Geometry check sheet. Reference: the model listing, model coordinates, mm. Face numbers are marked on the shaded views. A direction names the side the tool comes from. Give positions to 0.01 mm unless a question says otherwise; leave off trailing zeros. Write each loop counter-clockwise with the first axis right and the second up, starting at its lowest first coordinate (ties: lowest second). Pieces come first, ordered by that corner, then holes.
(1) Cross-section at A-A (y = -72.5). Record the boundary of the cut face in (x, z).
(2) Mould release check, pull along Z, two halves, no side actions. Record for the marked faces 1, 2 and 3: +Z half, -Z half, draft (parallel to the pull), parting line (faces both ways), or undercut.
(3) Cross-section at C-C (z = 7.75). Record the boundary of the cut face in (x, y), and give its area (3 significant figures).
(4) Thickness scan on line 1 along Z through (x, y) = (4, -66); line 2 along X through (y, z) = (8, 4.75); line 3 along X through (y, z) = (-44, 12.5). Record the ranges inside material, lowest first.
(5) Tool access check on the marked faces 4, 5 and 6. Record the directions out of +Z, -Z, +X, -X, +Y, -Y that give a thin tool (end or side, any length) a straight path to the whole face; none if there is none.
(6) Depth check by flat-ended pin: P1, Ø2, axis at y = -72.5, z = 15.5, coming from the -X side; P2, Ø5, axis at x = 2, y = -75, coming from the -Z side; P3, Ø4, axis at x = 7.5, z = 14, coming from the -Y side; P4, Ø8, axis at x = -2, z = 10.5, coming from the -Y side. Enter the tip coordinate at first touch or a pass-through.
(7) Cross-section at B-B (y = 0). Record the boundary of the cut face in (x, z).
(8) Cross-section at D-D (z = 17.75). Record the boundary of the cut face in (x, y).
```python
from build123d import *

# Parameters (mm, degrees)
SKETCH1_R           = 10
BOSS_EXTRUDE1_DEPTH = 20
SKETCH2_W           = 10
SKETCH2_H           = 35
CUT_EXTRUDE1_DEPTH  = 10


with BuildPart() as part:
    # Sketch1 → Boss-Extrude1 (new body)
    with BuildSketch(Plane.XY):
        with BuildLine():
            Line((5, -42), (10, -42))
            ThreePointArc((10, -42), (15.132819854, -26.12111797), (29.113715132, -17.009625152))
            ThreePointArc((29.113715132, -17.009625152), (42.376973847, 2.071419783), (25, 17.5))
            ThreePointArc((25, 17.5), (0, 10.405357444), (-25, 17.5))
            ThreePointArc((-25, 17.5), (-42.376973847, 2.071419783), (-29.113715132, -17.009625152))
            ThreePointArc((-29.113715132, -17.009625152), (-15.132819854, -26.12111797), (-10, -42))
            Line((-10, -42), (-5, -42))
            Line((-5, -42), (-5, -87))
            Line((-5, -87), (5, -87))
            Line((5, -87), (5, -42))
        make_face()
        with Locations((-25, 0)):
            Circle(SKETCH1_R, mode=Mode.SUBTRACT)
        with Locations(Location((25, 0, 0), (0, 0, 180))):
            Circle(SKETCH1_R, mode=Mode.SUBTRACT)
    extrude(amount=BOSS_EXTRUDE1_DEPTH)

    # Sketch2 → Cut-Extrude1 (cut)
    with BuildSketch(Plane(origin=(5, 0, 0), x_dir=(0, 0, -1), z_dir=(1, 0, 0))):
        with Locations((-10, -69.5)):
            Rectangle(SKETCH2_W, SKETCH2_H)
    extrude(amount=-CUT_EXTRUDE1_DEPTH, mode=Mode.SUBTRACT)


solid = part.part
```
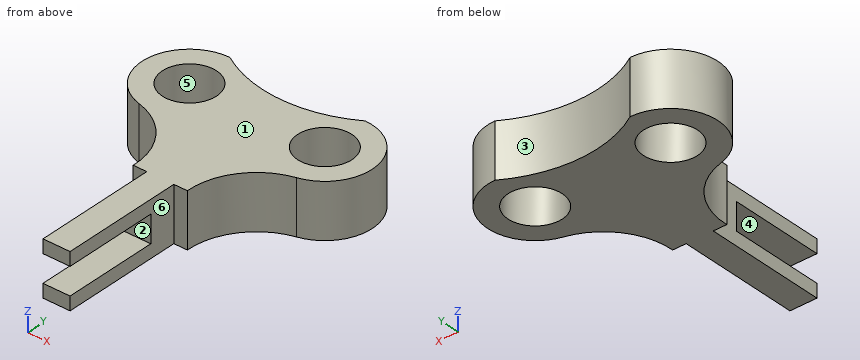
Reply:
1. outline: (-5, 0) - (5, 0) - (5, 5) - (-5, 5) - close; (-5, 15) - (5, 15) - (5, 20) - (-5, 20) - close
2. face 1: +Z half
2. face 2: undercut
2. face 3: draft
3. outline: (-29.11, -17.01) arc R25 cw to (-10, -42) - (-5, -42) - (-5, -52) - (5, -52) - (5, -42) - (10, -42) arc R25 cw to (29.11, -17.01) arc R17.5 ccw to (25, 17.5) arc R47.59 cw to (-25, 17.5) arc R17.5 ccw to start; hole circle Ø20 at (-25, 0); hole circle Ø20 at (25, 0)
3. area: 2,650 mm2
4. line 1: z = 0 to 5, 15 to 20
4. line 2: x = -40.56 to -31, -19 to 19, 31 to 40.56
4. line 3: x = -5 to 5
5. face 4: +X, -X, -Y
5. face 5: +Z, -Z
5. face 6: +Z, -Z, +X, -Y
6. P1: stops at x = -5
6. P2: stops at z = 0
6. P3: stops at y = -42
6. P4: stops at y = -52
7. outline: (-42.5, 0) - (-35, 0) - (-35, 20) - (-42.5, 20) - close; (-15, 0) - (15, 0) - (15, 20) - (-15, 20) - close; (35, 0) - (42.5, 0) - (42.5, 20) - (35, 20) - close
8. outline: (-29.11, -17.01) arc R25 cw to (-10, -42) - (-5, -42) - (-5, -87) - (5, -87) - (5, -42) - (10, -42) arc R25 cw to (29.11, -17.01) arc R17.5 ccw to (25, 17.5) arc R47.59 cw to (-25, 17.5) arc R17.5 ccw to start; hole circle Ø20 at (-25, 0); hole circle Ø20 at (25, 0)
